Part print with two shaded views. Sizes in mm from the minimum x, y, z corner. Give positions to 0.01 mm unless a question says otherwise; leave off trailing zeros. Order: outer loops, then holes, each group sorted by start corner. A loop starts at its lowest first (then second) coordinate and runs counter-clockwise, first axis right, second up. Notation, with made-up numbers: M 16,60 L 24,60 A26 ccw 24,95 Z; hole C 22,6 d7. An arc over 180 degrees is marked long. Return JSON: item names as keys, results as strings. Group by question number.
1. Slice it at B-B on y = 9.5. Give the number of separate pieces and of enclosed holes in the cut face.
2. Wall check: probe 1 along X at (y, z) = (2.25, 2.5) (1 decimal); probe 2 along X at (y, z) = (9.25, 2.5) (1 decimal); probe 3 along Z at (x, y) = (5, 9) (1 decimal). Give the ranges that are in metal, low to high. Write a range as [from, to].
3. Two-plate mould, pull along X, no slides. Class the marked faces 1, 2 and 3: released by +X, released by -X, zero draft, split by the parting line, or undercut.
4. Slice it at D-D on x = 2. List the corners of the cut face in (y, z).
5. Slice it at A-A on z = 3.5. List the corners of the cut face in (x, y), then the cut area to 3 significant figures.
6. Pin check, flat tip, straight feed: pin 1 (4.5 mm diameter, centred on x = 28.57, y = 5.57, fed in from -Z). Stop position of the tip, or through.
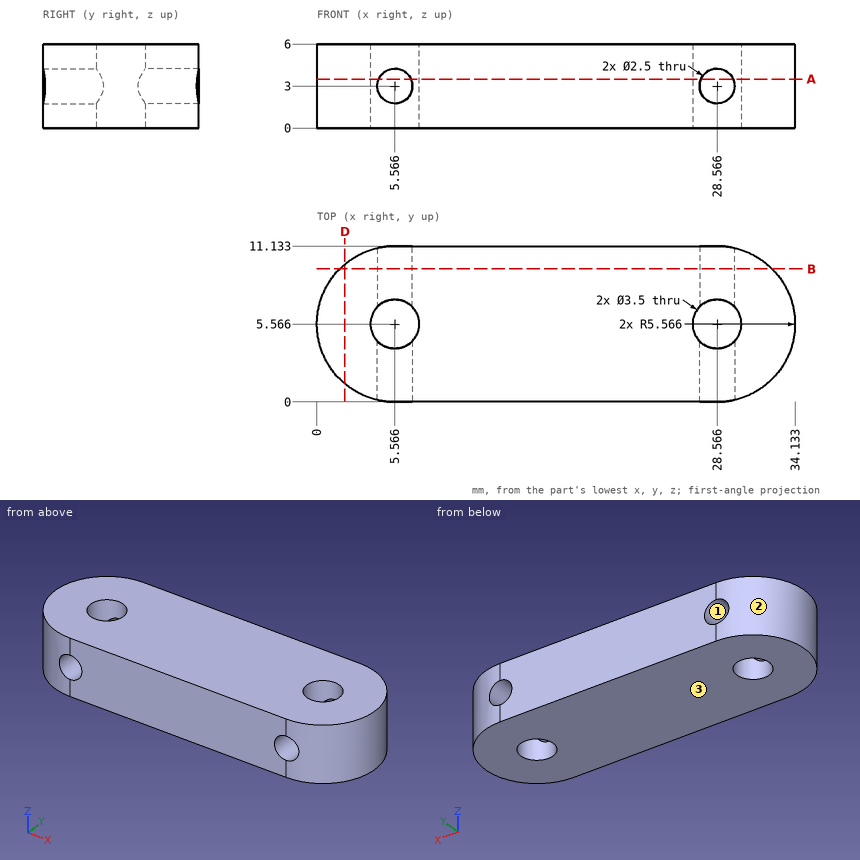
Result:
{
 "1": {"separate pieces": "1", "enclosed holes": "2"},
 "2": {"probe 1": "x = [1.1, 4.4], [6.7, 27.4], [29.7, 33]", "probe 2": "x = [1.4, 4.4], [6.7, 27.4], [29.7, 32.7]", "probe 3": "z = [0, 1.9], [4.1, 6]"},
 "3": {"face 1": "undercut", "face 2": "released by -X", "face 3": "zero draft"},
 "4": {"outline": "M 1.29,0 L 9.84,0 L 9.84,6 L 1.29,6 Z"},
 "5": {"outline": "M 4.42,0.12 L 4.42,4.24 A1.75 cw 4.42,6.89 L 4.42,11.01 A5.57 ccw Z; M 6.71,0 L 27.42,0 L 27.42,4.24 A1.75 cw 27.42,6.89 L 27.42,11.13 L 6.71,11.13 L 6.71,6.89 A1.75 cw 6.71,4.24 Z; M 29.71,0.12 A5.57 ccw 29.71,11.01 L 29.71,6.89 A1.75 cw 29.71,4.24 Z", "area": "298 mm2"},
 "6": {"pin 1": "stops at z = 0"}
}
